```python
from build123d import *
from build123d.topology import SkipClean

# Parameters (mm, degrees)
SKETCH1_R           = 10
SKETCH1_R_2         = 7.85
SKETCH1_R_3         = 3
BOSS_EXTRUDE3_DEPTH = 6
SKETCH2_R           = 7.85
CUT_EXTRUDE1_DEPTH  = 1
SKETCH3_R           = 6.85
CUT_EXTRUDE2_DEPTH  = 4.2
SKETCH5_R           = 7.85
SKETCH5_R_2         = 3
CUT_EXTRUDE3_DEPTH  = 1
SKETCH6_R           = 6.85
CUT_EXTRUDE4_DEPTH  = 4.2
CUT_EXTRUDE5_DEPTH  = 1.5
CUT_EXTRUDE6_START  = -1.5
CUT_EXTRUDE6_DEPTH  = 1.5
CUT_EXTRUDE9_DEPTH  = 1.75


with BuildPart() as part:
    # Sketch1 → Boss-Extrude3 (new body)
    # profile 1 of 5: a face of its own
    with BuildSketch(Plane(origin=(0, 0, 0), x_dir=(1, 0, 0), z_dir=(0, 1, 0))):
        with Locations((-120, 0)):
            Circle(SKETCH1_R)
        with Locations((-120, 0)):
            Circle(SKETCH1_R_2, mode=Mode.SUBTRACT)
    # profile 2 of 5: a face of its own
    with BuildSketch(Plane(origin=(0, 0, 0), x_dir=(1, 0, 0), z_dir=(0, 1, 0))):
        with Locations((-120, 0)):
            Circle(SKETCH1_R_2)
        with Locations(Location((-120, 0, 0), (0, 0, 270))):
            Circle(SKETCH1_R_3, mode=Mode.SUBTRACT)
    # profile 3 of 5: a face of its own
    with BuildSketch(Plane(origin=(0, 0, 0), x_dir=(1, 0, 0), z_dir=(0, 1, 0))):
        with BuildLine():
            ThreePointArc((-1.463415785, -9.892341191), (-10, 3.94e-07), (-1.463415006, 9.892341306))
            ThreePointArc((-1.463415006, 9.892341306), (-60.000000188, 5.585995813), (-118.536585366, 9.892341361))
            ThreePointArc((-118.536585366, 9.892341361), (-112.429196002, 6.533217188), (-110, 0))
            ThreePointArc((-110, 0), (-112.429196002, -6.533217188), (-118.536585366, -9.892341361))
            ThreePointArc((-118.536585366, -9.892341361), (-60.000000582, -5.585995813), (-1.463415785, -9.892341191))
        make_face()
    # profile 4 of 5: a face of its own
    with BuildSketch(Plane(origin=(0, 0, 0), x_dir=(1, 0, 0), z_dir=(0, 1, 0))):
        Circle(SKETCH1_R)
        Circle(SKETCH1_R_2, mode=Mode.SUBTRACT)
    # profile 5 of 5: a face of its own
    with BuildSketch(Plane(origin=(0, 0, 0), x_dir=(1, 0, 0), z_dir=(0, 1, 0))):
        Circle(SKETCH1_R_2)
        with Locations(Location((0, 0, 0), (0, 0, 270))):
            Circle(SKETCH1_R_3, mode=Mode.SUBTRACT)
    extrude(amount=BOSS_EXTRUDE3_DEPTH)

    # Sketch2 → Cut-Extrude1 (cut)
    with BuildSketch(Plane(origin=(0, 6, 0), x_dir=(1, 0, 0), z_dir=(0, 1, 0))):
        with Locations(Location((-120, 0, 0), (0, 0, 270))):
            Circle(SKETCH2_R)
    extrude(amount=-CUT_EXTRUDE1_DEPTH, mode=Mode.SUBTRACT)

    # Sketch3 → Cut-Extrude2 (cut)
    with BuildSketch(Plane(origin=(0, 5, 0), x_dir=(1, 0, 0), z_dir=(0, 1, 0))):
        with Locations(Location((-120, 0, 0), (0, 0, 270))):
            Circle(SKETCH3_R)
    extrude(amount=-CUT_EXTRUDE2_DEPTH, mode=Mode.SUBTRACT)

    # Sketch5 → Cut-Extrude3 (cut)
    with BuildSketch(Plane.XZ):
        with Locations(Location((0, 0, 0), (0, 0, 270))):
            Circle(SKETCH5_R)
        with Locations(Location((0, 0, 0), (0, 0, 270))):
            Circle(SKETCH5_R_2, mode=Mode.SUBTRACT)
    extrude(amount=-CUT_EXTRUDE3_DEPTH, mode=Mode.SUBTRACT)

    # Sketch6 → Cut-Extrude4 (cut)
    with BuildSketch(Plane.XZ.offset(-1)):
        with Locations(Location((0, 0, 0), (0, 0, 270))):
            Circle(SKETCH6_R)
    extrude(amount=-CUT_EXTRUDE4_DEPTH, mode=Mode.SUBTRACT)

    # Sketch7 → Cut-Extrude5 (cut)
    with BuildSketch(Plane.XZ):
        with BuildLine():
            ThreePointArc((-8.239471396, 5.666666667), (-5.29155752, 8.485247139), (-1.463414634, 9.892341361))
            ThreePointArc((-1.463414634, 9.892341361), (-60, 5.585995813), (-118.536585366, 9.892341361))
            ThreePointArc((-118.536585366, 9.892341361), (-114.70844248, 8.485247139), (-111.760528604, 5.666666667))
            ThreePointArc((-111.760528604, 5.666666667), (-109.968166246, 4.074693984), (-107.640792906, 3.5))
            Line((-107.640792906, 3.5), (-12.359207094, 3.5))
            ThreePointArc((-12.359207094, 3.5), (-10.031833754, 4.074693984), (-8.239471396, 5.666666667))
        make_face()
        with BuildLine():
            ThreePointArc((-118.536585366, -9.892341361), (-60, -5.585995813), (-1.463414634, -9.892341361))
            ThreePointArc((-1.463414634, -9.892341361), (-5.29155752, -8.485247139), (-8.239471396, -5.666666667))
            ThreePointArc((-8.239471396, -5.666666667), (-10.031833754, -4.074693984), (-12.359207094, -3.5))
            Line((-12.359207094, -3.5), (-107.640792906, -3.5))
            ThreePointArc((-107.640792906, -3.5), (-109.968166246, -4.074693984), (-111.760528604, -5.666666667))
            ThreePointArc((-111.760528604, -5.666666667), (-114.70844248, -8.485247139), (-118.536585366, -9.892341361))
        make_face()
    extrude(amount=-CUT_EXTRUDE5_DEPTH, mode=Mode.SUBTRACT)

    # Sketch8 → Cut-Extrude6 (cut)
    with SkipClean():  # the faces are left unmerged after this step: merging them gives an invalid solid
        with BuildSketch(Plane(origin=(0, 6, 0), x_dir=(1, 0, 0), z_dir=(0, 1, 0)).offset(CUT_EXTRUDE6_START)):
            with BuildLine():
                ThreePointArc((-1.463414634, 9.892341361), (-60, 5.585995813), (-118.536585366, 9.892341361))
                ThreePointArc((-118.536585366, 9.892341361), (-114.70844248, 8.485247139), (-111.760528604, 5.666666667))
                ThreePointArc((-111.760528604, 5.666666667), (-109.968166246, 4.074693984), (-107.640792906, 3.5))
                Line((-107.640792906, 3.5), (-12.359207094, 3.5))
                ThreePointArc((-12.359207094, 3.5), (-10.031833754, 4.074693984), (-8.239471396, 5.666666667))
                ThreePointArc((-8.239471396, 5.666666667), (-5.29155752, 8.485247139), (-1.463414634, 9.892341361))
            make_face()
            with BuildLine():
                Line((-12.359207094, -3.5), (-107.640792906, -3.5))
                ThreePointArc((-107.640792906, -3.5), (-109.968166246, -4.074693984), (-111.760528604, -5.666666667))
                ThreePointArc((-111.760528604, -5.666666667), (-114.70844248, -8.485247139), (-118.536585366, -9.892341361))
                ThreePointArc((-118.536585366, -9.892341361), (-60, -5.585995813), (-1.463414634, -9.892341361))
                ThreePointArc((-1.463414634, -9.892341361), (-5.29155752, -8.485247139), (-8.239471396, -5.666666667))
                ThreePointArc((-8.239471396, -5.666666667), (-10.031833754, -4.074693984), (-12.359207094, -3.5))
            make_face()
        extrude(amount=CUT_EXTRUDE6_DEPTH, mode=Mode.SUBTRACT)

    # Sketch10 → Cut-Extrude9 (cut)
    with BuildSketch(Plane.XZ):
        with BuildLine():
            ThreePointArc((-1.463414634, 9.892341361), (-60, 5.585995813), (-118.536585366, 9.892341361))
            ThreePointArc((-118.536585366, 9.892341361), (-114.70844248, 8.485247139), (-111.760528604, 5.666666667))
            ThreePointArc((-111.760528604, 5.666666667), (-109.968166246, 4.074693984), (-107.640792906, 3.5))
            Line((-107.640792906, 3.5), (-12.359207094, 3.5))
            ThreePointArc((-12.359207094, 3.5), (-10.031833754, 4.074693984), (-8.239471396, 5.666666667))
            ThreePointArc((-8.239471396, 5.666666667), (-5.29155752, 8.485247139), (-1.463414634, 9.892341361))
        make_face()
        with BuildLine():
            Line((-12.359207094, -3.5), (-107.640792906, -3.5))
            ThreePointArc((-107.640792906, -3.5), (-109.968166246, -4.074693984), (-111.760528604, -5.666666667))
            ThreePointArc((-111.760528604, -5.666666667), (-114.70844248, -8.485247139), (-118.536585366, -9.892341361))
            ThreePointArc((-118.536585366, -9.892341361), (-60, -5.585995813), (-1.463414634, -9.892341361))
            ThreePointArc((-1.463414634, -9.892341361), (-5.29155752, -8.485247139), (-8.239471396, -5.666666667))
            ThreePointArc((-8.239471396, -5.666666667), (-10.031833754, -4.074693984), (-12.359207094, -3.5))
        make_face()
    extrude(amount=-CUT_EXTRUDE9_DEPTH, mode=Mode.SUBTRACT)


solid = part.part
```
The listing builds one solid part. Answer for the finished solid, in the listing's coordinates (mm). A direction names the side the tool comes from. Give positions to 0.01 mm unless a question says otherwise; leave off trailing zeros. Loops run counter-clockwise (first coordinate to the right, second up) from the corner with the lowest first, then second, coordinate; pieces in that order, holes last. Notation, with made-up numbers: M 74,1 L 79,1 A22 ccw 79,32 Z; hole C 38,19.25 d7. An arc over 180 degrees is marked long. One line per item, written item: value.
1. Section B-B on x = 0 is taken. Determine the outline of the cut face in (y, z), plus the area to 3 significant figures.
Found:
outline: M 0,-10 L 6,-10 L 6,-3 L 5.2,-3 L 5.2,-6.85 L 1,-6.85 L 1,-7.85 L 0,-7.85 Z; M 0,7.85 L 1,7.85 L 1,6.85 L 5.2,6.85 L 5.2,3 L 6,3 L 6,10 L 0,10 Z
area: 42.0 mm^2
2. Section C-C on x = -15.5 is taken. Determine the outline of the cut face in (y, z).
Found:
outline: M 0,-3.5 L 1.75,-3.5 L 1.75,-8.07 L 4.5,-8.07 L 4.5,-3.5 L 6,-3.5 L 6,3.5 L 4.5,3.5 L 4.5,8.07 L 1.75,8.07 L 1.75,3.5 L 0,3.5 Z
3. For a pull along Z with two mould halves and no side action, classify faces 5 (the face through (-55, 6, -1)), 6 (the face through (-113.21, 2.93, -0.89)), 7 (the face through (-10.06, 5.24, -4.06)), 8 (the face through (-109.94, 5.24, 4.06)) as pulls with the +Z half, pulls with the -Z half, needs draft (parallel to the pull), parting line crosses it, or undercut.
Found:
face 5: needs draft
face 6: undercut
face 7: pulls with the -Z half
face 8: pulls with the +Z half
4. Each of these flat-tipped pins is pushed along its axis until it touches: P1, Ø3, axis at y = 4.5, z = -4, coming from the -X side; P2, Ø5, axis at x = -83, z = 6.5, coming from the -Y side; P3, Ø3, axis at x = -49, z = -5.5, coming from the +Y side; P4, Ø3.5, axis at x = 0, z = 0, coming from the -Y side. Where does it stop, or does it pass through?
Found:
P1: x = -129.68
P2: y = 1.75
P3: y = 4.5
P4: through
5. Find the intervals of material crossed by probe 1 along X at (y, z) = (5.45, 0); probe 2 along X at (y, z) = (4, 0); probe 3 along X at (y, z) = (1.4, 6.25), in increasing order.
Found:
probe 1: -130 to -127.85, -112.15 to -3, 3 to 10
probe 2: -130 to -126.85, -113.15 to -6.85, 6.85 to 10
probe 3: -127.81 to -122.8, -117.2 to -112.19, -7.81 to -2.8, 2.8 to 7.81
6. Section D-D on x = -109.5 is taken. Determine the outline of the cut face in (y, z).
Found:
outline: M 0,-3.86 L 1.75,-3.86 L 1.75,-8.66 L 4.5,-8.66 L 4.5,-3.86 L 6,-3.86 L 6,3.86 L 4.5,3.86 L 4.5,8.66 L 1.75,8.66 L 1.75,3.86 L 0,3.86 Z
7. For faces 1 (the face through (-61, 1.75, 5)), 2 (the face through (-110, 5.24, -4.09)), 3 (the face through (-10, 5.24, 4.09)), 4 (the face through (-61, 1.75, -5)), determine the directions among +Z, -Z, +X, -X, +Y, -Y from which every point of the face is accessible in a straight line to the end or side of a thin tool.
Found:
face 1: +Z, -Y
face 2: -Z, +Y
face 3: +Z, +Y
face 4: -Z, -Y
8. Section A-A on z = 0 is taken. Determine the outline of the cut face in (x, y), plus the area to 3 significant figures.
Found:
outline: M -130,0 L -123,0 L -123,0.8 L -126.85,0.8 L -126.85,5 L -127.85,5 L -127.85,6 L -130,6 Z; M -117,0 L -7.85,0 L -7.85,1 L -6.85,1 L -6.85,5.2 L -3,5.2 L -3,6 L -112.15,6 L -112.15,5 L -113.15,5 L -113.15,0.8 L -117,0.8 Z; M 3,5.2 L 6.85,5.2 L 6.85,1 L 7.85,1 L 7.85,0 L 10,0 L 10,6 L 3,6 Z
area: 684 mm^2
